CAD build for the part. Positions are in the model's coordinates, mm. Round coordinates to 2 decimals unless told otherwise and drop trailing zeros. Loops run counter-clockwise (first coordinate to the right, second up) from the corner with the lowest first, then second, coordinate; pieces in that order, holes last. Notation, with made-up numbers: M 8,-21 L 38,-21 A21 ccw 38,10 Z; hole C -25.75,59 d8. An arc over 180 degrees is marked long. Use a Markdown table: item, result. Add a question column.
(1) Band-saw the part on A-A, the plane x = 37.5. Write the cut outline in (y, z) (3 decimals).
(2) Band-saw the part on D-D, the plane z = 1.6. Write the cut outline in (x, y) (3 decimals), and give its area (3 significant figures).
(3) Band-saw the part on B-B, the plane y = 45.5. Write the cut outline in (x, z) (3 decimals).
(4) Band-saw the part on C-C, the plane x = 22. Write the cut outline in (y, z) (3 decimals), and give its area (3 significant figures).
(5) Wall check: L1, parallel to X at y = -18.5, z = 2.35; L2, parallel to Y at x = -39.5, z = 0.65; L3, parallel to Y at x = -51, z = 1.05 (3 decimals). Give the ranges that are in metal, low to high.
(6) Flat gauge pins, fed straight in: P1, Ø1.6, axis at x = 12, z = 1.5, coming from the -Y side; P2, Ø1, axis at x = -65.5, z = 2, coming from the -Y side (3 decimals); P3, Ø1.5, axis at y = 14.5, z = 2, coming from the -X side; P4, Ø12, axis at x = -27.5, y = -0.5, coming from the -Z side. Where does each tip first touch, or does it go through?
from build123d import *

# Parameters (mm, degrees)
SKETCH1_W           = 127
SKETCH1_H           = 177.8
BOSS_EXTRUDE1_DEPTH = 3.175
SKETCH3_W           = 63.5
SKETCH3_H           = 63.5
SKETCH3_W_2         = 109.22
SKETCH3_H_2         = 71.12
CUT_EXTRUDE2_DEPTH  = 4.175
BOSS_EXTRUDE2_DEPTH = 3.175
CUT_EXTRUDE3_REACH  = 5.175
SKETCH5_W           = 19.05
SKETCH5_H           = 12.7
CUT_EXTRUDE4_DEPTH  = 4.175


with BuildPart() as part:
    # Sketch1 → Boss-Extrude1 (new body)
    with BuildSketch(Plane.XY):
        Rectangle(SKETCH1_W, SKETCH1_H)
    extrude(amount=BOSS_EXTRUDE1_DEPTH)

    # Sketch3 → Cut-Extrude2 (cut, through all)
    with BuildSketch(Plane.XY.offset(3.175)):
        with Locations((0, 44.45)):
            Rectangle(SKETCH3_W, SKETCH3_H)
        with Locations((0, -27.94)):
            Rectangle(SKETCH3_W_2, SKETCH3_H_2)
    extrude(amount=-CUT_EXTRUDE2_DEPTH, mode=Mode.SUBTRACT)

    # Sketch4 → Boss-Extrude2 (add)
    with BuildSketch(Plane.XY.offset(3.175)):
        Polygon((-60.325, 92.075), (-66.675, 92.075), (-66.675, 85.725), (-66.675, 73.025), (-60.325, 73.025), (-60.325, 85.725), (-47.625, 85.725), (-47.625, 92.075), align=None)
        Polygon((60.325, 92.075), (66.675, 92.075), (66.675, 85.725), (66.675, 73.025), (60.325, 73.025), (60.325, 85.725), (47.625, 85.725), (47.625, 92.075), align=None)
    extrude(amount=-BOSS_EXTRUDE2_DEPTH)

    # Sketch5 → Cut-Extrude3 (cut, up to next)
    with BuildSketch(Plane.XY.offset(3.175), mode=Mode.PRIVATE) as cut_extrude3_sk1:
        with Locations((-53.975, -82.55)):
            Rectangle(SKETCH5_W, SKETCH5_H)
    cut_extrude3_tool1 = extrude(cut_extrude3_sk1.sketch, amount=-CUT_EXTRUDE3_REACH, mode=Mode.PRIVATE) & part.part
    add(cut_extrude3_tool1.solids().sort_by_distance((-53.975, -82.55, 3.175))[0], mode=Mode.SUBTRACT)
    # Sketch5 → Cut-Extrude3 (cut, up to next)
    with BuildSketch(Plane.XY.offset(3.175), mode=Mode.PRIVATE) as cut_extrude3_sk2:
        with Locations((53.975, -82.55)):
            Rectangle(SKETCH5_W, SKETCH5_H)
    cut_extrude3_tool2 = extrude(cut_extrude3_sk2.sketch, amount=-CUT_EXTRUDE3_REACH, mode=Mode.PRIVATE) & part.part
    add(cut_extrude3_tool2.solids().sort_by_distance((53.975, -82.55, 3.175))[0], mode=Mode.SUBTRACT)

    # Sketch6 → Cut-Extrude4 (cut, through all)
    with BuildSketch(Plane.XY.offset(3.175)):
        Polygon((-44.45, -76.2), (-44.45, -68.58), (44.45, -68.58), (44.45, -76.2), (44.45, -88.9), (-44.45, -88.9), align=None)
    extrude(amount=-CUT_EXTRUDE4_DEPTH, mode=Mode.SUBTRACT)


solid = part.part
Return value:
| question | item | result |
|---|---|---|
| 1 | outline | M -68.58,0 L -63.5,0 L -63.5,3.175 L -68.58,3.175 Z; M 7.62,0 L 88.9,0 L 88.9,3.175 L 7.62,3.175 Z |
| 2 | outline | M -66.675,73.025 L -63.5,73.025 L -63.5,-76.2 L -44.45,-76.2 L -44.45,-68.58 L 44.45,-68.58 L 44.45,-76.2 L 63.5,-76.2 L 63.5,73.025 L 66.675,73.025 L 66.675,92.075 L 47.625,92.075 L 47.625,88.9 L -47.625,88.9 L -47.625,92.075 L -66.675,92.075 Z; hole M -54.61,-63.5 L 54.61,-63.5 L 54.61,7.62 L -54.61,7.62 Z; hole M -31.75,12.7 L 31.75,12.7 L 31.75,76.2 L -31.75,76.2 Z |
| 2 | area | 8,710 mm^2 |
| 3 | outline | M -63.5,0 L -31.75,0 L -31.75,3.175 L -63.5,3.175 Z; M 31.75,0 L 63.5,0 L 63.5,3.175 L 31.75,3.175 Z |
| 4 | outline | M -68.58,0 L -63.5,0 L -63.5,3.175 L -68.58,3.175 Z; M 7.62,0 L 12.7,0 L 12.7,3.175 L 7.62,3.175 Z; M 76.2,0 L 88.9,0 L 88.9,3.175 L 76.2,3.175 Z |
| 4 | area | 72.6 mm^2 |
| 5 | L1 | -63.5 to -54.61, 54.61 to 63.5 |
| 5 | L2 | -68.58 to -63.5, 7.62 to 88.9 |
| 5 | L3 | -76.2 to -63.5, 7.62 to 92.075 |
| 6 | P1 | y = -68.58 |
| 6 | P2 | y = 73.025 |
| 6 | P3 | x = -63.5 |
| 6 | P4 | through |
